```python
from build123d import *

# Parameters (mm, degrees)
ENCLOSURE_TOP_SKETCH_W          = 74
ENCLOSURE_TOP_SKETCH_H          = 52
ENCLOSURE_TOP_FEATURE_DEPTH     = 4
SCREW_HOLES_SKETCH_R            = 1.6
SCREW_HOLES_FEATURE_DEPTH       = 46.398237851
CAMERA_LIGHT_HOLE_SKETCH_R      = 7.5
CAMERA_LIGHT_HOLE_SKETCH_W      = 20
CAMERA_LIGHT_HOLE_SKETCH_H      = 16
CAMERA_LIGHT_HOLE_SKETCH_W_2    = 10
CAMERA_LIGHT_HOLE_SKETCH_H_2    = 15
CAMERA_LIGHT_HOLE_SKETCH_W_3    = 12
CAMERA_LIGHT_HOLE_SKETCH_H_3    = 12
CAMERA_LIGHT_HOLE_FEATURE_DEPTH = 46.398237851
FILTER_COVER_SKETCH_R           = 9
FILTER_COVER_FEATURE_DEPTH      = 3.5
FILTER_CUT_SKETCH_R             = 6.5
FILTER_CUT_DEPTH                = 3.5
FILLET1_R                       = 1
FILLET2_R                       = 1
FILLET3_R                       = 1
FILLET4_R                       = 1
FILLET5_R                       = 1
FILLET6_R                       = 1


with BuildPart() as part:
    # Enclosure Top Sketch → Enclosure Top Feature (new body)
    with BuildSketch(Plane.XY):
        Rectangle(ENCLOSURE_TOP_SKETCH_W, ENCLOSURE_TOP_SKETCH_H)
    extrude(amount=ENCLOSURE_TOP_FEATURE_DEPTH)

    # Screw Holes Sketch → Screw Holes Feature (cut, through all)
    with BuildSketch(Plane.XY.offset(4)):
        with Locations((-31.1, 20.5)):
            Circle(SCREW_HOLES_SKETCH_R)
        with Locations((31.096, 20.5)):
            Circle(SCREW_HOLES_SKETCH_R)
        with Locations((31.1, -20.5)):
            Circle(SCREW_HOLES_SKETCH_R)
        with Locations((-31.096, -20.5)):
            Circle(SCREW_HOLES_SKETCH_R)
    extrude(amount=-SCREW_HOLES_FEATURE_DEPTH, mode=Mode.SUBTRACT)

    # Camera + Light Hole Sketch → Camera _ Light Hole Feature (cut, through all)
    with BuildSketch(Plane.XY.offset(4)):
        with Locations((-12, 0)):
            Circle(CAMERA_LIGHT_HOLE_SKETCH_R)
        with Locations((10, 0)):
            Rectangle(CAMERA_LIGHT_HOLE_SKETCH_W, CAMERA_LIGHT_HOLE_SKETCH_H)
        with Locations((32, 0)):
            Rectangle(CAMERA_LIGHT_HOLE_SKETCH_W_2, CAMERA_LIGHT_HOLE_SKETCH_H_2)
        with Locations((21.5, 17.714)):
            Rectangle(CAMERA_LIGHT_HOLE_SKETCH_W_3, CAMERA_LIGHT_HOLE_SKETCH_H_3)
    extrude(amount=-CAMERA_LIGHT_HOLE_FEATURE_DEPTH, mode=Mode.SUBTRACT)

    # Filter Cover Sketch → Filter Cover Feature (add)
    with BuildSketch(Plane(origin=(0, 0, 0), x_dir=(-1, 0, 0), z_dir=(0, 0, -1))):
        with Locations(Location((12, 0, 0), (0, 0, 180))):
            Circle(FILTER_COVER_SKETCH_R)
    extrude(amount=FILTER_COVER_FEATURE_DEPTH)

    # Filter Cut Sketch → Filter Cut (cut)
    with BuildSketch(Plane(origin=(0, 0, -3.5), x_dir=(-1, 0, 0), z_dir=(0, 0, -1))):
        with Locations((12, 0)):
            Circle(FILTER_CUT_SKETCH_R)
    extrude(amount=-FILTER_CUT_DEPTH, mode=Mode.SUBTRACT)

    # Fillet1
    fillet1_edges = [part.edges().sort_by_distance(p)[0] for p in [
        (0, 26, 0),
    ]]
    fillet(fillet1_edges, radius=FILLET1_R)

    # Fillet2
    fillet2_edges = [part.edges().sort_by_distance(p)[0] for p in [
        (-37, -0.5, 0),
        (-37, 25.707106781, 0.292893219),
        (-37, 26, 2.5),
    ]]
    fillet(fillet2_edges, radius=FILLET2_R)

    # Fillet3
    fillet3_edges = [part.edges().sort_by_distance(p)[0] for p in [
        (0.5, -26, 0),
        (-36.707106781, -26, 0.292893219),
        (-37, -26, 2.5),
    ]]
    fillet(fillet3_edges, radius=FILLET3_R)

    # Fillet4
    fillet4_edges = [part.edges().sort_by_distance(p)[0] for p in [
        (37, -16.25, 0),
        (37, -25.707106781, 0.292893219),
        (37, -26, 2.5),
    ]]
    fillet(fillet4_edges, radius=FILLET4_R)

    # Fillet5
    fillet5_edges = [part.edges().sort_by_distance(p)[0] for p in [
        (37, 25.707106781, 0.292893219),
        (37, 16.25, 0),
        (37, 26, 2.5),
    ]]
    fillet(fillet5_edges, radius=FILLET5_R)

    # Fillet6
    fillet6_edges = [part.edges().sort_by_distance(p)[0] for p in [
        (-21, 0, -3.5),
    ]]
    fillet(fillet6_edges, radius=FILLET6_R)


solid = part.part
```
The listing builds one solid part. Answer for the finished solid, in the listing's coordinates (mm). A direction names the side the tool comes from. Round coordinates to 2 decimals unless told otherwise and drop trailing zeros. Loops run counter-clockwise (first coordinate to the right, second up) from the corner with the lowest first, then second, coordinate; pieces in that order, holes last.
1) A cutting plane is placed at B-B on y = 0. Determine the outline of the cut face in (x, z), plus the area to 3 significant figures.
Outcome:
outline: (-37, 1) arc R1 ccw to (-36, 0) - (-21, 0) - (-21, -2.5) arc R1 ccw to (-20, -3.5) - (-18.5, -3.5) - (-18.5, 0) - (-19.5, 0) - (-19.5, 4) - (-37, 4) - close; (-5.5, -3.5) - (-4, -3.5) arc R1 ccw to (-3, -2.5) - (-3, 0) - (0, 0) - (0, 4) - (-4.5, 4) - (-4.5, 0) - (-5.5, 0) - close; (20, 0) - (27, 0) - (27, 4) - (20, 4) - close
area: 133 mm2
2) A cutting plane is placed at C-C on y = 12.5. Determine the outline of the cut face in (x, z).
Outcome:
outline: (-37, 1) arc R1 ccw to (-36, 0) - (15.5, 0) - (15.5, 4) - (-37, 4) - close; (27.5, 0) - (36, 0) arc R1 ccw to (37, 1) - (37, 4) - (27.5, 4) - close
3) Consider line 1 (Y direction, x = 6, z = 3); line 2 (Y direction, x = 31.1, z = 1); line 3 (X direction, y = 17, z = 3.25). Determine where each line is inside the solid, lowest interval first.
Outcome:
line 1: y = -26 to -8, 8 to 26
line 2: y = -26 to -22.1, -18.9 to -7.5, 7.5 to 18.9, 22.1 to 26
line 3: x = -37 to 15.5, 27.5 to 37
4) A cutting plane is placed at D-D on x = -31.1. Determine the outline of the cut face in (y, z), plus the area to 3 significant figures.
Outcome:
outline: (-26, 1) arc R1 ccw to (-25, 0) - (-22.1, 0) - (-22.1, 4) - (-26, 4) - close; (-18.9, 0) - (18.9, 0) - (18.9, 4) - (-18.9, 4) - close; (22.1, 0) - (25, 0) arc R1 ccw to (26, 1) - (26, 4) - (22.1, 4) - close
area: 182 mm2
5) For a pull along Y with two mould halves and no side action, classify faces 4 (the face through (-12, -7, -3.5)), 5 (the face through (-1, 26, 2)), 6 (the face through (-19.493, 0.33, 2.028)) as released by +Y, released by -Y, zero draft, split by the parting line, or undercut.
Outcome:
face 4: zero draft
face 5: released by +Y
face 6: undercut
6) Given P1, Ø13.5, axis at x = -12, y = 0, coming from the +Z side; P2, Ø1.2, axis at y = -1.5, z = 2, coming from the +X side; P3, Ø2.5, axis at x = 31.1, y = -20.5, coming from the -Z side; P4, Ø4, axis at x = -12.5, y = -20.5, coming from the -Z side, each flat-ended and moving along its own axis, determine where each tip first touches the part or whether it passes through.
Outcome:
P1: stops at z = 0
P2: stops at x = 27
P3: passes through
P4: stops at z = 0
7) A cutting plane is placed at A-A on x = 14.5. Determine the outline of the cut face in (y, z), plus the area to 3 significant figures.
Outcome:
outline: (-26, 1) arc R1 ccw to (-25, 0) - (-8, 0) - (-8, 4) - (-26, 4) - close; (8, 0) - (25, 0) arc R1 ccw to (26, 1) - (26, 4) - (8, 4) - close
area: 144 mm2
8) For faces 1 (the face through (37, -16, 2)), 2 (the face through (27.5, 18, 2)), 3 (the face through (27, 0, 2)), determine the directions among +Z, -Z, +X, -X, +Y, -Y from which every point of the face is accessible in a straight line to the end or side of a thin tool.
Outcome:
face 1: +Z, -Z, +X, +Y, -Y
face 2: +Z, -Z
face 3: +Z, -Z, +X
